```python
from build123d import *

# Parameters (mm, degrees)
CROQUIS1_W               = 90
CROQUIS1_H               = 76.2
CROQUIS1_R               = 4
SALIENTE_EXTRUIR1_DEPTH  = 0.47625
CROQUIS1_2_W             = 90
CROQUIS1_2_H             = 76.2
CROQUIS1_2_R             = 4
SALIENTE_EXTRUIR2_DEPTH  = 4.7625
CROQUIS3_W               = 90
CROQUIS3_H               = 4.7625
SALIENTE_EXTRUIR3_DEPTH  = 4.445
CROQUIS5_W               = 90
CROQUIS5_H               = 4.7625
SALIENTE_EXTRUIR4_DEPTH  = 4.445
CROQUIS6_W               = 4.7625
CROQUIS6_H               = 85.09
SALIENTE_EXTRUIR5_DEPTH  = 5
CROQUIS7_W               = 4.7625
CROQUIS7_H               = 85.09
SALIENTE_EXTRUIR6_DEPTH  = 5
CROQUIS8_W               = 100
CROQUIS8_H               = 4.7625
SALIENTE_EXTRUIR7_DEPTH  = 4.445
CROQUIS9_W               = 100
CROQUIS9_H               = 4.7625
SALIENTE_EXTRUIR8_DEPTH  = 4.445
CROQUIS10_W              = 4.7625
CROQUIS10_H              = 93.98
SALIENTE_EXTRUIR9_DEPTH  = 5
CROQUIS12_W              = 4.7625
CROQUIS12_H              = 93.98
SALIENTE_EXTRUIR10_DEPTH = 5


with BuildPart() as part:
    # Croquis1 → Saliente-Extruir1 (new body)
    with BuildSketch(Plane.XY):
        with Locations((45, 38.1)):
            Rectangle(CROQUIS1_W, CROQUIS1_H)
        with Locations((45, 38.1)):
            Circle(CROQUIS1_R, mode=Mode.SUBTRACT)
        with Locations((10, 9.95)):
            Circle(CROQUIS1_R, mode=Mode.SUBTRACT)
        with Locations((10, 66.25)):
            Circle(CROQUIS1_R, mode=Mode.SUBTRACT)
        with Locations((80, 66.25)):
            Circle(CROQUIS1_R, mode=Mode.SUBTRACT)
        with Locations((80, 9.95)):
            Circle(CROQUIS1_R, mode=Mode.SUBTRACT)
        with Locations((45, 66.25)):
            Circle(CROQUIS1_R, mode=Mode.SUBTRACT)
        with Locations((10, 38.1)):
            Circle(CROQUIS1_R, mode=Mode.SUBTRACT)
        with Locations((80, 38.1)):
            Circle(CROQUIS1_R, mode=Mode.SUBTRACT)
        with Locations((45, 9.95)):
            Circle(CROQUIS1_R, mode=Mode.SUBTRACT)
    extrude(amount=SALIENTE_EXTRUIR1_DEPTH)

    # Croquis1<2> → Saliente-Extruir2 (add)
    with BuildSketch(Plane.XY):
        with Locations((45, 38.1)):
            Rectangle(CROQUIS1_2_W, CROQUIS1_2_H)
        with Locations((45, 38.1)):
            Circle(CROQUIS1_2_R, mode=Mode.SUBTRACT)
        with Locations((10, 9.95)):
            Circle(CROQUIS1_2_R, mode=Mode.SUBTRACT)
        with Locations((10, 66.25)):
            Circle(CROQUIS1_2_R, mode=Mode.SUBTRACT)
        with Locations((80, 66.25)):
            Circle(CROQUIS1_2_R, mode=Mode.SUBTRACT)
        with Locations((80, 9.95)):
            Circle(CROQUIS1_2_R, mode=Mode.SUBTRACT)
        with Locations((45, 66.25)):
            Circle(CROQUIS1_2_R, mode=Mode.SUBTRACT)
        with Locations((10, 38.1)):
            Circle(CROQUIS1_2_R, mode=Mode.SUBTRACT)
        with Locations((80, 38.1)):
            Circle(CROQUIS1_2_R, mode=Mode.SUBTRACT)
        with Locations((45, 9.95)):
            Circle(CROQUIS1_2_R, mode=Mode.SUBTRACT)
    extrude(amount=SALIENTE_EXTRUIR2_DEPTH)

    # Croquis3 → Saliente-Extruir3 (add)
    with BuildSketch(Plane.XZ):
        with Locations((45, 2.38125)):
            Rectangle(CROQUIS3_W, CROQUIS3_H)
    extrude(amount=SALIENTE_EXTRUIR3_DEPTH)

    # Croquis5 → Saliente-Extruir4 (add)
    with BuildSketch(Plane(origin=(0, 76.2, 0), x_dir=(1, 0, 0), z_dir=(0, 1, 0))):
        with Locations((45, -2.38125)):
            Rectangle(CROQUIS5_W, CROQUIS5_H)
    extrude(amount=SALIENTE_EXTRUIR4_DEPTH)

    # Croquis6 → Saliente-Extruir5 (add)
    with BuildSketch(Plane.ZY):
        with Locations((2.38125, 38.1)):
            Rectangle(CROQUIS6_W, CROQUIS6_H)
    extrude(amount=SALIENTE_EXTRUIR5_DEPTH)

    # Croquis7 → Saliente-Extruir6 (add)
    with BuildSketch(Plane(origin=(90, 0, 0), x_dir=(0, 0, -1), z_dir=(1, 0, 0))):
        with Locations((-2.38125, 38.1)):
            Rectangle(CROQUIS7_W, CROQUIS7_H)
    extrude(amount=SALIENTE_EXTRUIR6_DEPTH)

    # Croquis8 → Saliente-Extruir7 (add)
    with BuildSketch(Plane.XZ.offset(4.445)):
        with Locations((45, 2.38125)):
            Rectangle(CROQUIS8_W, CROQUIS8_H)
    extrude(amount=SALIENTE_EXTRUIR7_DEPTH)

    # Croquis9 → Saliente-Extruir8 (add)
    with BuildSketch(Plane(origin=(0, 80.645, 0), x_dir=(1, 0, 0), z_dir=(0, 1, 0))):
        with Locations((45, -2.38125)):
            Rectangle(CROQUIS9_W, CROQUIS9_H)
    extrude(amount=SALIENTE_EXTRUIR8_DEPTH)

    # Croquis10 → Saliente-Extruir9 (add)
    with BuildSketch(Plane(origin=(95, 0, 0), x_dir=(0, 0, -1), z_dir=(1, 0, 0))):
        with Locations((-2.38125, 38.1)):
            Rectangle(CROQUIS10_W, CROQUIS10_H)
    extrude(amount=SALIENTE_EXTRUIR9_DEPTH)

    # Croquis12 → Saliente-Extruir10 (add)
    with BuildSketch(Plane.ZY.offset(5)):
        with Locations((2.38125, 38.1)):
            Rectangle(CROQUIS12_W, CROQUIS12_H)
    extrude(amount=SALIENTE_EXTRUIR10_DEPTH)


solid = part.part
```
Input: part model. Units: mm. Frame: model coordinates. Give positions to 0.01 mm unless a question says otherwise; leave off trailing zeros. Order: outer loops, then holes, each group sorted by start corner. A loop starts at its lowest first (then second) coordinate and runs counter-clockwise, first axis right, second up. Notation, with made-up numbers: M 2.25,19 L 19.25,19 A21 ccw 19.25,29 Z; hole C 69,42 d8. An arc over 180 degrees is marked long. Return JSON: item names as keys, results as strings.
1) Line query: L1, parallel to Y at x = 10, z = 2.5; L2, parallel to X at y = 38.5, z = 3.45; L3, parallel to Y at x = 42, z = 3.45. Output: solid intervals per line, ascending. Write a range as [from, to].
Taken from the geometry:
{"L1": "y = [-8.89, 5.95], [13.95, 34.1], [42.1, 62.25], [70.25, 85.09]", "L2": "x = [-10, 6.02], [13.98, 41.02], [48.98, 76.02], [83.98, 100]", "L3": "y = [-8.89, 7.3], [12.6, 35.45], [40.75, 63.6], [68.9, 85.09]"}
2) Mould query, pull axis Y, two halves, no side actions, for faces 1 (the face through (79.133, 62.345, 2.348)), 2 (the face through (46, 27, 4.762)), 3 (the face through (44.133, 62.345, 2.348)), 4 (the face through (46, 85.09, 2)). Classes: released by +Y, released by -Y, zero draft, split by the parting line, or undercut.
Taken from the geometry:
{"face 1": "undercut", "face 2": "zero draft", "face 3": "undercut", "face 4": "released by +Y"}
3) Section query C-C on z = 1.15. Count the separate pieces of the cut face and the enclosed holes in it, and give its area (3 significant figures).
Taken from the geometry:
{"separate pieces": "1", "enclosed holes": "9", "area": "9,890 mm2"}
4) Contact query for a flat-ended pin moving along its axis: pin 1 (10.5 mm diameter, centred on x = 80, y = 38.1, fed in from +Z). Output: stop coordinate, or through.
Taken from the geometry:
{"pin 1": "stops at z = 4.76"}
5) Section query B-B on x = 80. Output: boundary loops of the cut face in (y, z).
Taken from the geometry:
{"outline": "M -8.89,0 L 5.95,0 L 5.95,4.76 L -8.89,4.76 Z; M 13.95,0 L 34.1,0 L 34.1,4.76 L 13.95,4.76 Z; M 42.1,0 L 62.25,0 L 62.25,4.76 L 42.1,4.76 Z; M 70.25,0 L 85.09,0 L 85.09,4.76 L 70.25,4.76 Z"}
6) Section query A-A on y = 9.95. Output: boundary loops of the cut face in (x, z).
Taken from the geometry:
{"outline": "M -10,0 L 6,0 L 6,4.76 L -10,4.76 Z; M 14,0 L 41,0 L 41,4.76 L 14,4.76 Z; M 49,0 L 76,0 L 76,4.76 L 49,4.76 Z; M 84,0 L 100,0 L 100,4.76 L 84,4.76 Z"}
